from build123d import *

# Parameters (mm, degrees)
SKETCH_1_R         = 13
EXTRUDE_1138_DEPTH = 14
CHAMFER_1_SIZE     = 4


with BuildPart() as part:
    # 草图1 → Extrude 1138 (new body)
    with BuildSketch(Plane.XY):
        Polygon((135, 155), (155, 135), (155, -155), (-135, -155), (-155, -135), (-155, 155), align=None)
        with Locations((-113.13708499, -113.13708499)):
            Circle(SKETCH_1_R, mode=Mode.SUBTRACT)
        with Locations((-78.524110604, -61.919012055)):
            Circle(SKETCH_1_R, mode=Mode.SUBTRACT)
        with Locations((78.524110604, 61.919012055)):
            Circle(SKETCH_1_R, mode=Mode.SUBTRACT)
        with Locations((113.13708499, 113.13708499)):
            Circle(SKETCH_1_R, mode=Mode.SUBTRACT)
        with Locations((-70.710678119, 70.710678119)):
            Circle(SKETCH_1_R, mode=Mode.SUBTRACT)
        with Locations((-113.13708499, 113.13708499)):
            Circle(SKETCH_1_R, mode=Mode.SUBTRACT)
        with Locations(Location((70.710678119, -70.710678119, 0), (0, 0, 180))):
            Circle(SKETCH_1_R, mode=Mode.SUBTRACT)
        with Locations(Location((113.13708499, -113.13708499, 0), (0, 0, 180))):
            Circle(SKETCH_1_R, mode=Mode.SUBTRACT)
        Circle(SKETCH_1_R, mode=Mode.SUBTRACT)
    extrude(amount=EXTRUDE_1138_DEPTH)

    # 倒角1
    chamfer_1_edges = [part.edges().sort_by_distance(p)[0] for p in [
        (10, -155, 14),
        (155, -10, 14),
        (145, 145, 14),
        (-126.13708499, -113.13708499, 0),
        (-126.13708499, -113.13708499, 14),
        (-10, 155, 14),
        (-91.524110604, -61.919012055, 0),
        (-91.524110604, -61.919012055, 14),
        (65.524110604, 61.919012055, 0),
        (65.524110604, 61.919012055, 14),
        (100.13708499, 113.13708499, 0),
        (100.13708499, 113.13708499, 14),
        (-83.710678119, 70.710678119, 0),
        (-83.710678119, 70.710678119, 14),
        (-126.13708499, 113.13708499, 0),
        (-126.13708499, 113.13708499, 14),
        (83.710678119, -70.710678119, 0),
        (83.710678119, -70.710678119, 14),
        (-155, 10, 14),
        (-13, 0, 0),
        (-13, 0, 14),
        (126.13708499, -113.13708499, 0),
        (126.13708499, -113.13708499, 14),
        (-10, 155, 0),
        (145, 145, 0),
        (155, -10, 0),
        (-145, -145, 14),
        (10, -155, 0),
        (-145, -145, 0),
        (-155, 10, 0),
    ]]
    chamfer(chamfer_1_edges, length=CHAMFER_1_SIZE)


solid = part.part
The listing builds one solid part. Answer for the finished solid, in the listing's coordinates (mm). Give positions to 0.01 mm unless a question says otherwise; leave off trailing zeros. Order: outer loops, then holes, each group sorted by start corner. A loop starts at its lowest first (then second) coordinate and runs counter-clockwise, first axis right, second up. Notation, with made-up numbers: (-7, 66.5) - (23, 66.5) arc R15 ccw to (23, 92.5) - close; hole circle Ø9 at (89.25, 2). An arc over 180 degrees is marked (long way). Use one line per item in the form item = value.
1) Find section C-C on z = 6.5. Give the number of separate pieces and of enclosed holes in the cut face, and give its area (3 significant figures).
Verdict:
separate_pieces = 1
enclosed_holes = 9
area = 90,900 mm^2
2) This flat-tipped pin is pushed along its axis until it touches: pin 1 (10 mm diameter, centred on x = -107, y = -119.5, fed in from +Z). Where does it stop, or does it pass through?
Verdict:
pin_1 = 10.84
3) The mould has two halves that part along X. Classify faces 1 (the flat face through (-143.426, -143.706, 12.028)), 2 (the flat face through (143.426, 143.706, 12.028)), 3 (the cylindrical face through (76.83, 74.81, 6.96)), 4 (the cylindrical face through (-122.72, 121.92, 6.96)): released by +X, released by -X, zero draft, split by the parting line, or undercut.
Verdict:
face_1 = released by -X
face_2 = released by +X
face_3 = undercut
face_4 = undercut
4) Find section A-A on y = 0. Determine the outline of the cut face in (x, z), and give its area (3 significant figures).
Verdict:
outline = (-155, 4) - (-151, 0) - (-17, 0) - (-13, 4) - (-13, 10) - (-17, 14) - (-151, 14) - (-155, 10) - close; (13, 4) - (17, 0) - (151, 0) - (155, 4) - (155, 10) - (151, 14) - (17, 14) - (13, 10) - close
area = 3,910 mm^2
5) Consider probe 1 along X at (y, z) = (126, 12.25); probe 2 along X at (y, z) = (-59, 11); probe 3 along Y at (x, z) = (103.5, 4). Determine where each line is inside the solid, lowest interval first. Write a range as [from, to].
Verdict:
probe_1 = [-152.75, -121.33], [-104.95, 104.95], [121.33, 152.75]
probe_2 = [-154, -92.22], [-64.83, 63.04], [78.38, 154]
probe_3 = [-155, -121.86], [-104.41, 104.41], [121.86, 155]
